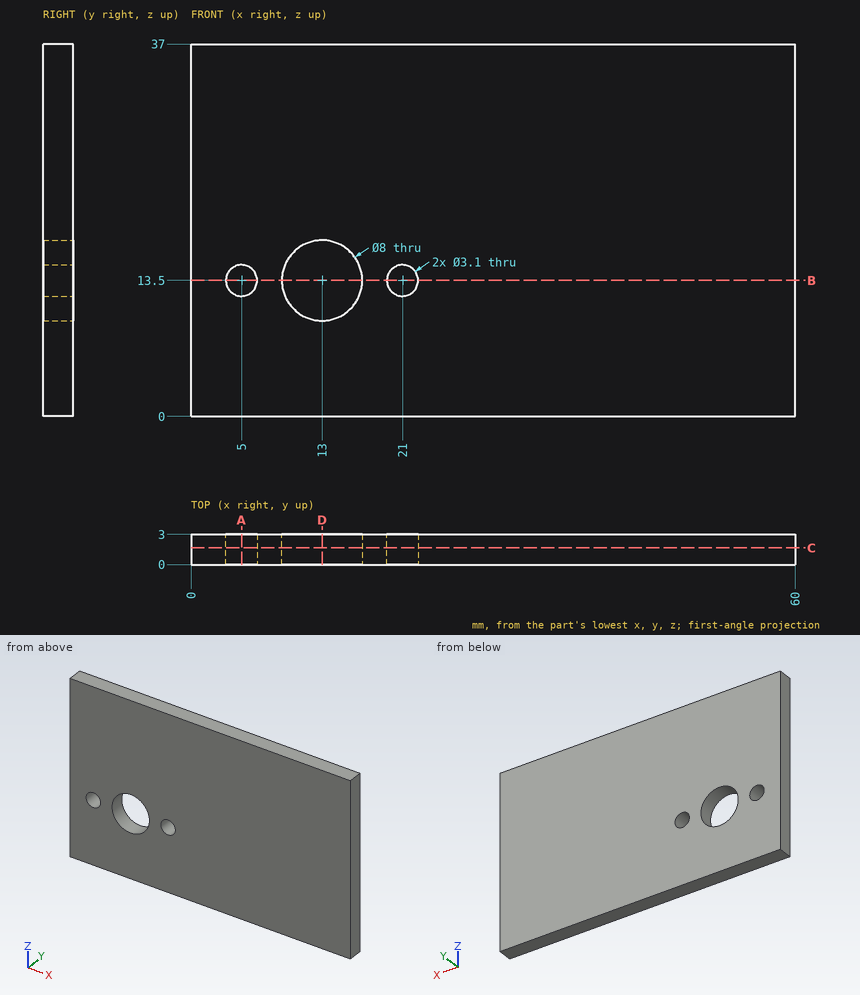
Could you check a few things on this drawing? It's one solid part, dimensions in mm from its lowest x, y, z. Give positions to 0.01 mm unless a question says otherwise; leave off trailing zeros. Write each loop counter-clockwise with the first axis right and the second up, starting at its lowest first coordinate (ties: lowest second). Pieces come first, ordered by that corner, then holes.
(1) If I drill on L1, parallel to Z at x = 5, y = 2.2; L2, parallel to X at y = 1.95, z = 10.5, over which ranges is the centre line in solid material (lowest first)?
Output values:
L1: z = 0 to 11.95, 15.05 to 37
L2: x = 0 to 10.35, 15.65 to 60
(2) Imagine slicing it at B-B, the plane z = 13.5. Write out the boundary of the cut face in (x, y).
Output values:
outline: (0, 0) - (3.45, 0) - (3.45, 3) - (0, 3) - close; (6.55, 0) - (9, 0) - (9, 3) - (6.55, 3) - close; (17, 0) - (19.45, 0) - (19.45, 3) - (17, 3) - close; (22.55, 0) - (60, 0) - (60, 3) - (22.55, 3) - close
(3) Imagine slicing it at C-C, the plane y = 1.65. Write out the boundary of the cut face in (x, z), and give its area (3 significant figures).
Output values:
outline: (0, 0) - (60, 0) - (60, 37) - (0, 37) - close; hole circle Ø3.1 at (5, 13.5); hole circle Ø8 at (13, 13.5); hole circle Ø3.1 at (21, 13.5)
area: 2,150 mm2
(4) Imagine slicing it at A-A, the plane x = 5. Write out the boundary of the cut face in (y, z), and give its area (3 significant figures).
Output values:
outline: (0, 0) - (3, 0) - (3, 11.95) - (0, 11.95) - close; (0, 15.05) - (3, 15.05) - (3, 37) - (0, 37) - close
area: 102 mm2
(5) Imagine slicing it at D-D, the plane x = 13. Write out the boundary of the cut face in (y, z), and give its area (3 significant figures).
Output values:
outline: (0, 0) - (3, 0) - (3, 9.5) - (0, 9.5) - close; (0, 17.5) - (3, 17.5) - (3, 37) - (0, 37) - close
area: 87.0 mm2
